The listing builds one solid part. Answer for the finished solid, in the listing's coordinates (mm). A direction names the side the tool comes from. Round coordinates to 2 decimals unless told otherwise and drop trailing zeros. Loops run counter-clockwise (first coordinate to the right, second up) from the corner with the lowest first, then second, coordinate; pieces in that order, holes last. Notation, with made-up numbers: (-32, -28.75) -> (4, -28.75) arc R20 ccw to (4, -22.75) -> close; hole circle Ø3 at (-13, 83). An arc over 180 degrees is marked (long way). Use a Markdown table: item, result. Add a question column.
Q1. Consider line 1 (Z direction, x = 0, y = -13.5) (3 decimals); line 2 (Z direction, x = 0, y = -16); line 3 (Y direction, x = -6, z = -118.5). Determine where each line is inside the solid, lowest interval first.
Q2. Section B-B on x = 0 is taken. Give the vertices of the cut face in (y, z) (3 decimals).
Q3. Section A-A on z = -133.5 is taken. Give the vertices of the cut face in (x, y).
Q4. Which of the six approach directions +Z, -Z, +X, -X, +Y, -Y give full straight-line access (tool end or side, diameter ignored) to faces 1 (the flat face through (0.3, 5.3, 0)), 2 (the flat face through (0, 5.08, 3)), 3 (the cylindrical face through (-0.3, -16.2, -55.1))?
Q5. For a pull along Y with two mould halves and no side action, classify faces 4 (the flat face through (0, -7, 5.08)), 5 (the flat face through (0, 16.637, -88)), 6 (the flat face through (0, -5.08, 3)) as released by +Y, released by -Y, zero draft, split by the parting line, or undercut.
Q6. Section D-D on x = 19 is taken. Give the vertices of the cut face in (y, z).
Q7. Section C-C on y = -10 is taken. Give the vertices of the cut face in (x, z).
Q8. Given pin 1 Ø6 at (y, z) = (-9.5, -108.5) entering from -X; pin 2 Ø10 at (y, z) = (6.5, -110) entering from +X; pin 3 Ø5 at (y, z) = (10.5, -157.5) entering from +X, each flat-ended and moving along its own axis, determine where each tip first touches the part or whether it passes through.
from build123d import *

# Parameters (mm, degrees)
BOSS_EXTRUDE1_DEPTH = 177.8
BOSS_EXTRUDE2_DEPTH = 5.08
SKETCH5_R           = 3.683
CUT_EXTRUDE2_DEPTH  = 4.191
SKETCH6_R           = 2.286
CUT_EXTRUDE3_DEPTH  = 6.731
CUT_EXTRUDE5_DEPTH  = 5.08


with BuildPart() as part:
    # Sketch1 → Boss-Extrude1 (new body)
    with BuildSketch(Plane.XY):
        with BuildLine():
            ThreePointArc((-24.13, 0), (-20.74503307, 8.17203307), (-12.573, 11.557))
            Line((-12.573, 11.557), (12.573, 11.557))
            ThreePointArc((12.573, 11.557), (20.74503307, 8.17203307), (24.13, 0))
            Line((24.13, 0), (26.67, 0))
            ThreePointArc((26.67, 0), (21.797135519, 11.764135519), (10.033, 16.637))
            Line((10.033, 16.637), (-10.033, 16.637))
            ThreePointArc((-10.033, 16.637), (-21.797135519, 11.764135519), (-26.67, 0))
            Line((-26.67, 0), (-24.13, 0))
        make_face()
        with BuildLine():
            ThreePointArc((-12.573, -11.557), (-20.74503307, -8.17203307), (-24.13, 0))
            Line((-24.13, 0), (-26.67, 0))
            ThreePointArc((-26.67, 0), (-21.797135519, -11.764135519), (-10.033, -16.637))
            Line((-10.033, -16.637), (10.033, -16.637))
            ThreePointArc((10.033, -16.637), (21.797135519, -11.764135519), (26.67, 0))
            Line((26.67, 0), (24.13, 0))
            ThreePointArc((24.13, 0), (20.74503307, -8.17203307), (12.573, -11.557))
            Line((12.573, -11.557), (-12.573, -11.557))
        make_face()
    extrude(amount=-BOSS_EXTRUDE1_DEPTH)

    # Sketch3 → Boss-Extrude2 (add)
    with BuildSketch(Plane.XY):
        with BuildLine():
            Line((-10.033, 16.637), (10.033, 16.637))
            ThreePointArc((10.033, 16.637), (26.67, 0), (10.033, -16.637))
            Line((10.033, -16.637), (-10.033, -16.637))
            ThreePointArc((-10.033, -16.637), (-26.67, 0), (-10.033, 16.637))
        make_face()
    extrude(amount=BOSS_EXTRUDE2_DEPTH)

    # Sketch5 → Cut-Extrude2 (cut)
    with BuildSketch(Plane(origin=(0, -11.557, 0), x_dir=(1, 0, 0), z_dir=(0, 1, 0))):
        with Locations((0, 119.888)):
            Circle(SKETCH5_R)
        with Locations((0, 52.832)):
            Circle(SKETCH5_R)
    extrude(amount=-CUT_EXTRUDE2_DEPTH, mode=Mode.SUBTRACT)

    # Sketch6 → Cut-Extrude3 (cut)
    with BuildSketch(Plane(origin=(0, -11.557, 0), x_dir=(1, 0, 0), z_dir=(0, 1, 0))):
        with Locations((0, 119.888)):
            Circle(SKETCH6_R)
        with Locations((0, 52.832)):
            Circle(SKETCH6_R)
    extrude(amount=-CUT_EXTRUDE3_DEPTH, mode=Mode.SUBTRACT)

    # Sketch7 → Cut-Extrude5 (cut)
    with BuildSketch(Plane.XY.offset(5.08)):
        with BuildLine():
            Line((-3.175, 5.08), (3.175, 5.08))
            ThreePointArc((3.175, 5.08), (8.255, 0), (3.175, -5.08))
            Line((3.175, -5.08), (-3.175, -5.08))
            ThreePointArc((-3.175, -5.08), (-8.255, 0), (-3.175, 5.08))
        make_face()
    extrude(amount=-CUT_EXTRUDE5_DEPTH, mode=Mode.SUBTRACT)


solid = part.part
Checked values:
| question | item | result |
|---|---|---|
| 1 | line 1 | z = -177.8 to -123.571, -116.205 to -56.515, -49.149 to 5.08 |
| 1 | line 2 | z = -177.8 to -122.17, -117.6 to -55.12, -50.55 to 5.08 |
| 1 | line 3 | y = -16.64 to -11.56, 11.56 to 16.64 |
| 2 | outline | (-16.637, -177.8) -> (-11.557, -177.8) -> (-11.557, -123.571) -> (-15.748, -123.571) -> (-15.748, -122.174) -> (-16.637, -122.174) -> close; (-16.637, -117.602) -> (-15.748, -117.602) -> (-15.748, -116.205) -> (-11.557, -116.205) -> (-11.557, -56.515) -> (-15.748, -56.515) -> (-15.748, -55.118) -> (-16.637, -55.118) -> close; (-16.637, -50.546) -> (-15.748, -50.546) -> (-15.748, -49.149) -> (-11.557, -49.149) -> (-11.557, 0) -> (-5.08, 0) -> (-5.08, 5.08) -> (-16.637, 5.08) -> close; (5.08, 0) -> (11.557, 0) -> (11.557, -177.8) -> (16.637, -177.8) -> (16.637, 5.08) -> (5.08, 5.08) -> close |
| 3 | outline | (-10.03, -16.64) -> (10.03, -16.64) arc R16.64 ccw to (10.03, 16.64) -> (-10.03, 16.64) arc R16.64 ccw to start; hole (-12.57, -11.56) -> (12.57, -11.56) arc R11.56 ccw to (12.57, 11.56) -> (-12.57, 11.56) arc R11.56 ccw to start |
| 4 | face 1 | -Z |
| 4 | face 2 | +Z, -Z |
| 4 | face 3 | -Y |
| 5 | face 4 | zero draft |
| 5 | face 5 | released by +Y |
| 5 | face 6 | undercut |
| 6 | outline | (-14.01, -177.8) -> (-9.61, -177.8) -> (-9.61, 0) -> (9.61, 0) -> (9.61, -177.8) -> (14.01, -177.8) -> (14.01, 5.08) -> (-14.01, 5.08) -> close |
| 7 | outline | (-23.33, -177.8) -> (-18.37, -177.8) -> (-18.37, 0) -> (18.37, 0) -> (18.37, -177.8) -> (23.33, -177.8) -> (23.33, 5.08) -> (-23.33, 5.08) -> close |
| 8 | pin 1 | stops at x = -25.35 |
| 8 | pin 2 | stops at x = 26.6 |
| 8 | pin 3 | stops at x = 24.62 |
